Read the model definition and answer for the solid it produces. Units are mm, in the model's axes. A direction names the side the tool comes from. Give positions to 0.01 mm unless a question says otherwise; leave off trailing zeros. Loops run counter-clockwise (first coordinate to the right, second up) from the corner with the lowest first, then second, coordinate; pieces in that order, holes last. Notation, with made-up numbers: (38.5, 84.25) -> (96.5, 84.25) arc R19 cw to (96.5, 109.25) -> close; hole circle Ø9 at (-14, 67). An arc over 180 degrees is marked (long way). Write each question's results on one line, items separated by ' | '. Start each with the question number.
Item 1: Section A-A on z = 0 is taken. Write down the section's boundary in (x, y) (3 decimals), and give its area (3 significant figures).
Item 2: Determine the mould class of faces 4 (the flat face through (39, 0, 0)), 5 (the flat face through (25, 5, 0)), 6 (the cylindrical face through (25, -6, 0)) for opening direction Z: +Z half, -Z half, draft (parallel to the pull), parting line (faces both ways), or undercut.
Item 3: Which of the six approach directions +Z, -Z, +X, -X, +Y, -Y give full straight-line access (tool end or side, diameter ignored) to faces 1 (the cylindrical face through (46.88, 3.18, -1.19)), 2 (the cylindrical face through (44.92, -2.05, 0.46)), 3 (the flat face through (0, 0, 0))?
Item 4: Section B-B on x = 40 is taken. Write down the section's boundary in (y, z), and give its area (3 significant figures).
Item 5: Section C-C on y = 0 is taken. Write down the section's boundary in (x, z), and give its area (3 significant figures).
Item 6: Find the intervals of material crossed by line 1 (X direction, y = 3.35, z = 0); line 2 (Y direction, x = 33, z = 5); line 3 (X direction, y = 3, z = -1), in increasing order.
Item 7: This flat-tipped pin is pushed along its axis until it touches: P1, Ø3, axis at x = 46.5, z = 0, coming from the +Y side (3 decimals). Where does it stop, or does it pass through?
Item 8: Section D-D on x = 46.5 is taken. Write down the section's boundary in (y, z) (3 decimals), and give its area (3 significant figures).
```python
from build123d import *

# Parameters (mm, degrees)
SKETCH1_R                   = 6
BOSS_EXTRUDE1_DEPTH         = 51
CUT_EXTRUDE1_START          = -12
SKETCH2_R                   = 2.1
CUT_EXTRUDE1_DEPTH          = 12
M3_TAPPED_HOLE1_D           = 2.5
M3_TAPPED_HOLE1_DEPTH       = 6
M3_TAPPED_HOLE1_CSINK_D     = 3.05
M3_TAPPED_HOLE1_CSINK_ANGLE = 90
M3_TAPPED_HOLE1_TIP         = 0.751075774
CUT_EXTRUDE2_REACH          = 41.912


with BuildPart() as part:
    # Sketch1 → Boss-Extrude1 (new body)
    with BuildSketch(Plane(origin=(0, 0, 0), x_dir=(0, 0, -1), z_dir=(1, 0, 0))):
        Circle(SKETCH1_R)
    extrude(amount=BOSS_EXTRUDE1_DEPTH)

    # Sketch2 → Cut-Extrude1 (cut)
    with BuildSketch(Plane(origin=(51, 0, 0), x_dir=(0, 0, -1), z_dir=(1, 0, 0)).offset(CUT_EXTRUDE1_START)):
        Circle(SKETCH2_R)
        with BuildLine():
            Line((-3.31662479, 5), (3.31662479, 5))
            ThreePointArc((3.31662479, 5), (0, 6), (-3.31662479, 5))
        make_face()
    extrude(amount=CUT_EXTRUDE1_DEPTH, mode=Mode.SUBTRACT)

    # M3 Tapped Hole1
    with Locations(Plane(origin=(46.5, 5, 0), x_dir=(0, 0, 1), z_dir=(0, 1, 0))):
        with Locations((0, 0)):
            CounterSinkHole(M3_TAPPED_HOLE1_D / 2, M3_TAPPED_HOLE1_CSINK_D / 2, depth=M3_TAPPED_HOLE1_DEPTH, counter_sink_angle=M3_TAPPED_HOLE1_CSINK_ANGLE)
            with Locations((0, 0, -(M3_TAPPED_HOLE1_DEPTH + M3_TAPPED_HOLE1_TIP / 2))):  # 118° drill point
                Cone(0, M3_TAPPED_HOLE1_D / 2, M3_TAPPED_HOLE1_TIP, mode=Mode.SUBTRACT)

    # Sketch7 → Cut-Extrude2 (cut, up to next)
    with BuildSketch(Plane(origin=(39, 0, 0), x_dir=(0, 0, -1), z_dir=(1, 0, 0)), mode=Mode.PRIVATE) as cut_extrude2_sk1:
        with BuildLine():
            Line((-3.31662479, 5), (3.31662479, 5))
            ThreePointArc((3.31662479, 5), (0, 6), (-3.31662479, 5))
        make_face()
    cut_extrude2_tool1 = extrude(cut_extrude2_sk1.sketch, amount=-CUT_EXTRUDE2_REACH, mode=Mode.PRIVATE) & part.part
    add(cut_extrude2_tool1.solids().sort_by_distance((39, 5.403002, 0))[0], mode=Mode.SUBTRACT)


solid = part.part
```
Findings:
1) outline: (0, -6) -> (51, -6) -> (51, -2.1) -> (39, -2.1) -> (39, 2.1) -> (45.25, 2.1) -> (45.25, 4.725) -> (44.975, 5) -> (0, 5) -> close; (47.75, 2.1) -> (51, 2.1) -> (51, 5) -> (48.025, 5) -> (47.75, 4.725) -> close | area: 503 mm2
2) face 4: undercut | face 5: draft | face 6: parting line
3) face 1: +Y | face 2: +X | face 3: +Z, -Z, -X, +Y, -Y
4) outline: (5, -3.32) -> (5, 3.32) arc R6 ccw (long way) to start; hole circle Ø4.2 at (0, 0) | area: 94.7 mm2
5) outline: (0, -6) -> (51, -6) -> (51, -2.1) -> (39, -2.1) -> (39, 2.1) -> (51, 2.1) -> (51, 6) -> (0, 6) -> close | area: 562 mm2
6) line 1: 0 to 45.25, 47.75 to 51 | line 2: -3.32 to 3.32 | line 3: 0 to 45.75, 47.25 to 51
7) P1: y = 4.975
8) outline: (1.687, -1.25) arc R2.1 cw (long way) to (1.687, 1.25) -> (4.725, 1.25) -> (5, 1.525) -> (5, 3.317) arc R6 ccw (long way) to (5, -3.317) -> (5, -1.525) -> (4.725, -1.25) -> close | area: 87.1 mm2
